Source: CAD feature listing. Evaluate the final solid. Frame: model axes, mm. A direction names the side the tool comes from. Give positions to 0.01 mm unless a question says otherwise; leave off trailing zeros. Write each loop counter-clockwise with the first axis right and the second up, starting at its lowest first coordinate (ties: lowest second). Pieces come first, ordered by that corner, then holes. Notation, with made-up numbers: (38, 81) -> (79, 81) arc R10 ccw to (79, 90) -> close; hole circle Ø9 at (58, 17.25). An arc over 180 degrees is marked (long way). Write item = value, one per line.
from build123d import *

# Parameters (mm, degrees)
BASPROSKE_W     = 12
BASPROSKE_H     = 16.25
TOOTHCUT_DEPTH  = 26.925373671
TEETHCUTS_COUNT = 24
TEETHCUTS_ANGLE = 345
BORSKE_R        = 12
BORE_DEPTH      = 50.0000508
SKETCH_1_R      = 12
SKETCH_1_R_2    = 9.25
EXTRUDE_1_DEPTH = 12
EXTRUDE_2_DEPTH = 12


with BuildPart() as part:
    # BasProSke → Base-Revolve (revolve)
    with BuildSketch(Plane(origin=(0, 0, 0), x_dir=(1, 0, 0), z_dir=(0, 1, 0)), mode=Mode.PRIVATE) as base_revolve_sk:
        with Locations((6, 8.125)):
            Rectangle(BASPROSKE_W, BASPROSKE_H)
    revolve(base_revolve_sk.sketch.rotate(Axis((-10, 0, 0), (1, 0, 0)), 180), axis=Axis((-10, 0, 0), (1, 0, 0)))

    # TooCutSke → ToothCut (cut, through all)
    with BuildSketch(Plane(origin=(0, 0, 0), x_dir=(0, 0, -1), z_dir=(1, 0, 0))):
        with BuildLine():
            ThreePointArc((0.600427448, 13.423077856), (0, 13.4365), (-0.600427448, 13.423077856))
            ThreePointArc((-0.600427448, 13.423077856), (-1.021266982, 14.875437681), (-1.791844283, 16.176462507))
            ThreePointArc((-1.791844283, 16.176462507), (0, 16.2754), (1.791844283, 16.176462507))
            ThreePointArc((1.791844283, 16.176462507), (1.021266982, 14.875437681), (0.600427448, 13.423077856))
        make_face()
    toothcut = extrude(amount=TOOTHCUT_DEPTH, mode=Mode.SUBTRACT)

    # TeethCuts: ToothCut ×24 about axis
    teethcuts_axis = Axis((-10, 0, 0), (1, 0, 0))
    for i in range(1, TEETHCUTS_COUNT):
        add(toothcut.rotate(teethcuts_axis, i * TEETHCUTS_ANGLE / (TEETHCUTS_COUNT - 1)), mode=Mode.SUBTRACT)

    # BorSke → Bore (cut, symmetric)
    with BuildSketch(Plane(origin=(0, 0, 0), x_dir=(0, 0, -1), z_dir=(1, 0, 0))):
        with Locations(Location((0, 0, 0), (0, 0, 180))):
            Circle(BORSKE_R)
    extrude(amount=BORE_DEPTH, both=True, mode=Mode.SUBTRACT)

    # 草图1 → 凸台-拉伸1 (add, through all)
    with BuildSketch(Plane.ZY):
        Circle(SKETCH_1_R)
        Circle(SKETCH_1_R_2, mode=Mode.SUBTRACT)
    extrude(amount=-EXTRUDE_1_DEPTH)

    # 草图2 → 凸台-拉伸2 (add, through all)
    with BuildSketch(Plane.ZY):
        with BuildLine():
            Line((-7.5, 5.414101957), (-7.5, -5.414101957))
            ThreePointArc((-7.5, -5.414101957), (-9.25, 0), (-7.5, 5.414101957))
        make_face()
        with BuildLine():
            Line((7.5, 5.414101957), (7.5, -5.414101957))
            ThreePointArc((7.5, -5.414101957), (9.25, 0), (7.5, 5.414101957))
        make_face()
    extrude(amount=-EXTRUDE_2_DEPTH)


solid = part.part
(1) Material intervals for line 1 (Y direction, x = 2.25, z = 14.5); line 2 (Y direction, x = 4, z = -9.5); line 3 (Y direction, x = 9.5, z = 1), sorted ascending.
Values follow:
line_1 = -6.58 to -5.18, -2.88 to -0.87, 0.87 to 2.88, 5.18 to 6.58
line_2 = -13.05 to -10.6, -9.5 to 9.5, 10.6 to 13.05
line_3 = -14.83 to -9.2, 9.2 to 14.83
(2) Section query A-A (z = 14). Return loops of the section in (x, y).
Values follow:
outline = (0, -6.59) -> (12, -6.59) -> (12, -4.76) -> (0, -4.76) -> close; (0, -2.92) -> (12, -2.92) -> (12, -0.72) -> (0, -0.72) -> close; (0, 0.72) -> (12, 0.72) -> (12, 2.92) -> (0, 2.92) -> close; (0, 4.76) -> (12, 4.76) -> (12, 6.59) -> (0, 6.59) -> close
(3) Access query for faces 4 (the face through (5.916, -4.814, 14.076)), 5 (the face through (5.916, 4.814, -14.076)), 6 (the face through (5.92, 11.63, -6.73)). Directions: +Z, -Z, +X, -X, +Y, -Y. A direction counts if a zero-diameter tool reaches every point of the face in a straight line with its end or side. Return the directions, or none.
Values follow:
face_4 = +Z, +X, -X
face_5 = -Z, +X, -X
face_6 = +X, -X
(4) First-contact query: pin 1 (6 mm diameter, centred on x = 7, z = 3, fed in from -Y); pin 2 (6 mm diameter, centred on x = 7, z = 12, fed in from -Y); pin 3 (1 mm diameter, centred on x = 9.5, y = -1, fed in from -Z). Flat tips, straight axial feed; report the tip coordinate or a pass-through.
Values follow:
pin_1 = -16.15
pin_2 = -13.1
pin_3 = -15.77
(5) Pull-direction query (Y, two-part tool) for faces 1 (the face through (5.9, 9.5, 9.5)), 2 (the face through (5.92, -12.38, 8.33)), 3 (the face through (12, 0, -8)); classes: pulls with the +Y half, pulls with the -Y half, needs draft (parallel to the pull), parting line crosses it, or undercut.
Values follow:
face_1 = undercut
face_2 = pulls with the -Y half
face_3 = needs draft
